Geometry check sheet. Reference: the model listing, model coordinates, mm. A direction names the side the tool comes from. Give positions to 0.01 mm unless a question says otherwise; leave off trailing zeros. Order: outer loops, then holes, each group sorted by start corner. A loop starts at its lowest first (then second) coordinate and runs counter-clockwise, first axis right, second up. Notation, with made-up numbers: M 50.5,78 L 95.5,78 A16 cw 95.5,82 Z; hole C 59.25,32.25 d11. An arc over 180 degrees is marked long. Put each result on its own line as item: value. Start each with the question number.
Q1. Mould release check, pull along X, two halves, no side actions. Record for faces 4 (the flat face through (15, 135.537, 61)), 5 (the cylindrical face through (-21.701, 177.542, -23.666)), 6 (the cylindrical face through (16.91, 190.49, -26.53)): +X half, -X half, draft (parallel to the pull), parting line (faces both ways), or undercut.
Q2. Section check B-B on z = 0. Record the cut outline in (x, y), then the cut area to 3 significant figures.
Q3. Go/stop test with flat-tipped pins: pin 1 (8 mm diameter, centred on x = 5.5, z = 47, fed in from -Y); pin 2 (2 mm diameter, centred on x = -16, y = 142, fed in from +Z); pin 3 (19 mm diameter, centred on x = 13, z = -11.5, fed in from +Y). Record where each tip stops, or that it passes through.
Q4. Access from +Z, -Z, +X, -X, +Y, -Y to the whole of each face (thin tool, end or side, straight path). Record for faces 1 (the flat face through (26, 189.043, 0)), 2 (the conical face through (-4.45, 157.96, -33.86)), 3 (the flat face through (28, 182.693, 17)).
Q5. Material ranges on L1, parallel to X at y = 190, z = 0; L2, parallel to X at y = 180, z = 0; L3, parallel to Y at x = -33, z = 18, recorded low to high.
Q6. Section check D-D on y = 174. Record the cut outline in (x, z).
Q7. Section check C-C on y = 185.5. Record the cut outline in (x, z), then the cut area to 3 significant figures.
Q8. Section check A-A on x = 0. Record the cut outline in (y, z).
```python
from build123d import *


# Read off the part's stored shape, not the designer's step: Shell1
with BuildPart() as part:
    # Sketch1 → Revolve1 (revolve)
    with BuildSketch(Plane.XY, mode=Mode.PRIVATE) as revolve1_sk:
        with BuildLine():
            Line((0, 0), (55.850610629, 0))
            ThreePointArc((55.850610629, 0), (64.83086675, 3.719743879), (68.550610629, 12.7))
            Line((68.550610629, 12.7), (68.550610629, 135.537090781))
            ThreePointArc((68.550610629, 135.537090781), (67.07437947, 141.479902659), (62.988876295, 146.041145392))
            Line((62.988876295, 146.041145392), (36.426242146, 164.092378593))
            ThreePointArc((36.426242146, 164.092378593), (33.255344861, 167.632513451), (32.109591896, 172.244930881))
            Line((32.109591896, 172.244930881), (32.109591896, 182.693006016))
            Line((32.109591896, 182.693006016), (37.812538782, 182.693006016))
            Line((37.812538782, 182.693006016), (37.812538782, 191.889991998))
            Line((37.812538782, 191.889991998), (0, 191.889991998))
            Line((0, 191.889991998), (0, 0))
        make_face()
    revolve(revolve1_sk.sketch.rotate(Axis((0, 191.889991998, 0), (0, -1, 0)), 90), axis=Axis((0, 191.889991998, 0), (0, -1, 0)))

    # Shell1 outline → Shell1 (revolve, cut)
    with BuildSketch(Plane.XY):
        with BuildLine():
            Line((68.550610629, 135.537090781), (62.200610629, 135.537090781))
            ThreePointArc((62.200610629, 135.537090781), (61.462495049, 138.50849672), (59.419743462, 140.789118087))
            Line((59.419743462, 140.789118087), (32.857109313, 158.840351287))
            ThreePointArc((32.857109313, 158.840351287), (27.643460441, 164.661107512), (25.759591896, 172.244930881))
            Line((25.759591896, 172.244930881), (25.759591896, 189.043006016))
            Line((25.759591896, 189.043006016), (31.462538782, 189.043006016))
            Line((31.462538782, 189.043006016), (31.462538782, 191.889991998))
            Line((31.462538782, 191.889991998), (0, 191.889991998))
            Line((0, 191.889991998), (0, 0))
            Line((0, 0), (55.850610629, 0))
            ThreePointArc((55.850610629, 0), (64.83086675, 3.719743879), (68.550610629, 12.7))
            Line((68.550610629, 12.7), (68.550610629, 135.537090781))
        make_face()
    revolve(axis=Axis((0, 0, 0), (0, 1, 0)), mode=Mode.SUBTRACT)


solid = part.part
```
Results found:
1. face 4: draft
1. face 5: parting line
1. face 6: undercut
2. outline: M -68.55,135.54 L -62.2,135.54 A6.35 cw -59.42,140.79 L -32.86,158.84 A16.21 ccw -25.76,172.24 L -25.76,189.04 L -31.46,189.04 L -31.46,191.89 L -37.81,191.89 L -37.81,182.69 L -32.11,182.69 L -32.11,172.24 A9.86 cw -36.43,164.09 L -62.99,146.04 A12.7 ccw Z; M 25.76,172.24 A16.21 ccw 32.86,158.84 L 59.42,140.79 A6.35 cw 62.2,135.54 L 68.55,135.54 A12.7 ccw 62.99,146.04 L 36.43,164.09 A9.86 cw 32.11,172.24 L 32.11,182.69 L 37.81,182.69 L 37.81,191.89 L 31.46,191.89 L 31.46,189.04 L 25.76,189.04 Z
2. area: 1,010 mm^2
3. pin 1: stops at y = 146.29
3. pin 2: stops at z = 65.44
3. pin 3: stops at y = 189.04
4. face 1: +Y
4. face 2: -Y
4. face 3: none
5. L1: x = -37.81 to -31.46, 31.46 to 37.81
5. L2: x = -32.11 to -25.76, 25.76 to 32.11
5. L3: y = 155.62 to 163.3, 182.69 to 191.89
6. outline: C 0,0 d64.22; hole C 0,0 d51.52
7. outline: C 0,0 d75.63; hole C 0,0 d51.52
7. area: 2,410 mm^2
8. outline: M 135.54,-68.55 A12.7 ccw 146.04,-62.99 L 164.09,-36.43 A9.86 cw 172.24,-32.11 L 182.69,-32.11 L 182.69,-37.81 L 191.89,-37.81 L 191.89,-31.46 L 189.04,-31.46 L 189.04,-25.76 L 172.24,-25.76 A16.21 ccw 158.84,-32.86 L 140.79,-59.42 A6.35 cw 135.54,-62.2 Z; M 135.54,62.2 A6.35 cw 140.79,59.42 L 158.84,32.86 A16.21 ccw 172.24,25.76 L 189.04,25.76 L 189.04,31.46 L 191.89,31.46 L 191.89,37.81 L 182.69,37.81 L 182.69,32.11 L 172.24,32.11 A9.86 cw 164.09,36.43 L 146.04,62.99 A12.7 ccw 135.54,68.55 Z
